Source: CAD feature listing. Evaluate the final solid. Frame: model axes, mm. Face numbers are marked on the shaded views. Round coordinates to 2 decimals unless told otherwise and drop trailing zeros. Order: outer loops, then holes, each group sorted by start corner. A loop starts at its lowest first (then second) coordinate and runs counter-clockwise, first axis right, second up. Notation, with made-up numbers: (65, 2.5) -> (111, 2.5) arc R10 cw to (111, 7.5) -> close; hole circle Ø8 at (74.25, 30.25). An arc over 180 degrees is marked (long way). One line per item, written item: value. Start each with the question number.
1) Section C-C (z = 64). Return the cut outline in (x, y), and give its area (3 significant figures).
2) Mould query, pull axis Y, two halves, no side actions, for the marked faces 1, 2 and 3. Classes: pulls with the +Y half, pulls with the -Y half, needs draft (parallel to the pull), parting line crosses it, or undercut.
3) Ray query, L1, parallel to Y at x = 0, z = 51; L2, parallel to Z at x = 19, y = -5.5; L3, parallel to Y at x = 23, z = 30. Return the intervals inside material, ascending.
4) Section A-A (y = 0). Return the cut outline in (x, z), and give its area (3 significant figures).
5) Pin query (flat end, axial travel): P1, Ø10, axis at x = 6, y = 11.5, coming from the +Z side; P2, Ø3, axis at x = -16.5, z = 51.5, coming from the +Y side; P3, Ø4, axis at y = 9.5, z = 15.5, coming from the -X side. Return the tip coordinate at first contact, or that it passes through.
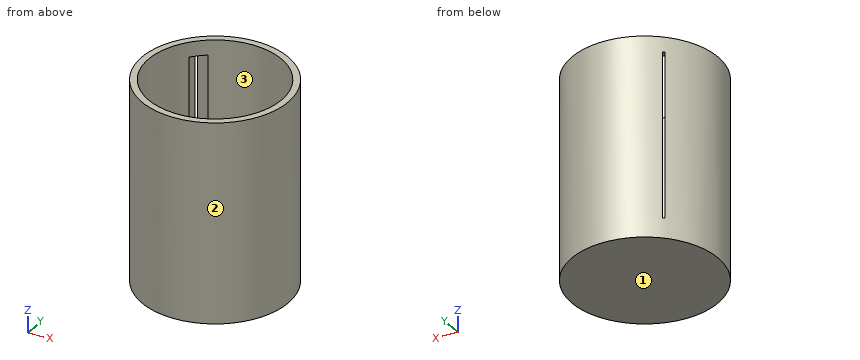
```python
from build123d import *

# Parameters (mm, degrees)
F0_R     = 30
F1_DEPTH = 3
F0_R_2   = 33
F2_DEPTH = 90
F3_W     = 9.444052
F3_H     = 74.371448
F4_DEPTH = 24.5


with BuildPart() as f1:
    # F0 (on Top) → F1 (new body)
    with BuildSketch(Plane.XY):
        Circle(F0_R)
    extrude(amount=F1_DEPTH)

    # F0 (on Top) → F2 (join)
    with BuildSketch(Plane.XY):
        Circle(F0_R_2)
        Circle(F0_R, mode=Mode.SUBTRACT)
    extrude(amount=F2_DEPTH)

    # F3 (on Front) → F4 (cut)
    with BuildSketch(Plane.XZ):
        with Locations((-18.13293, 46.117877)):
            Rectangle(F3_W, F3_H)
    extrude(amount=-F4_DEPTH, mode=Mode.SUBTRACT)


solid = f1.part
```
Findings:
1. outline: (-22.85, 19.43) -> (-22.85, 23.8) arc R33 ccw (long way) to (-22.11, 24.5) -> (-17.31, 24.5) arc R30 cw (long way) to start
1. area: 581 mm2
2. face 1: needs draft
2. face 2: parting line crosses it
2. face 3: undercut
3. L1: -33 to -30, 30 to 33
3. L2: 0 to 3
3. L3: -23.66 to -19.26, 19.26 to 23.66
4. outline: (-33, 0) -> (33, 0) -> (33, 90) -> (30, 90) -> (30, 3) -> (-30, 3) -> (-30, 90) -> (-33, 90) -> close
4. area: 720 mm2
5. P1: z = 3
5. P2: y = 29.39
5. P3: x = -32.14
